from build123d import *

# Parameters (mm, degrees)
SKETCH1_W           = 130
SKETCH1_H           = 15
BOSS_EXTRUDE1_DEPTH = 6
SKETCH2_W           = 90
SKETCH2_H           = 15
BOSS_EXTRUDE2_DEPTH = 22
CUT_EXTRUDE1_REACH  = 134.699
SKETCH3_R           = 3.5
CUT_EXTRUDE2_REACH  = 134.699
SKETCH4_R           = 12.5
CUT_EXTRUDE3_REACH  = 135.825
SKETCH5_R           = 1.625
SKETCH6_R           = 3.5
CUT_EXTRUDE4_DEPTH  = 25.5
FILLET1_R           = 3
FILLET3_R           = 1.5


with BuildPart() as part:
    # Sketch1 → Boss-Extrude1 (new body)
    with BuildSketch(Plane(origin=(0, 0, 0), x_dir=(1, 0, 0), z_dir=(0, 1, 0))):
        with Locations((65, 7.5)):
            Rectangle(SKETCH1_W, SKETCH1_H)
    extrude(amount=BOSS_EXTRUDE1_DEPTH)

    # Sketch2 → Boss-Extrude2 (add)
    with BuildSketch(Plane(origin=(0, 6, 0), x_dir=(1, 0, 0), z_dir=(0, 1, 0))):
        with Locations((65, 7.5)):
            Rectangle(SKETCH2_W, SKETCH2_H)
    extrude(amount=BOSS_EXTRUDE2_DEPTH)

    # Sketch3 → Cut-Extrude1 (cut, up to next)
    with BuildSketch(Plane(origin=(0, 6, 0), x_dir=(1, 0, 0), z_dir=(0, 1, 0)), mode=Mode.PRIVATE) as cut_extrude1_sk1:
        with Locations(Location((10, 7.5, 0), (0, 0, 270))):
            Circle(SKETCH3_R)
    cut_extrude1_tool1 = extrude(cut_extrude1_sk1.sketch, amount=-CUT_EXTRUDE1_REACH, mode=Mode.PRIVATE) & part.part
    # Sketch3 → Cut-Extrude1 (cut, up to next)
    with BuildSketch(Plane(origin=(0, 6, 0), x_dir=(1, 0, 0), z_dir=(0, 1, 0)), mode=Mode.PRIVATE) as cut_extrude1_sk2:
        with Locations(Location((120, 7.5, 0), (0, 0, 270))):
            Circle(SKETCH3_R)
    cut_extrude1_tool2 = extrude(cut_extrude1_sk2.sketch, amount=-CUT_EXTRUDE1_REACH, mode=Mode.PRIVATE) & part.part
    add(cut_extrude1_tool1.solids().sort_by_distance((10, 6, -7.5))[0], mode=Mode.SUBTRACT)
    add(cut_extrude1_tool2.solids().sort_by_distance((120, 6, -7.5))[0], mode=Mode.SUBTRACT)

    # Sketch4 → Cut-Extrude2 (cut, up to next)
    with BuildSketch(Plane(origin=(0, 6, 0), x_dir=(1, 0, 0), z_dir=(0, 1, 0)), mode=Mode.PRIVATE) as cut_extrude2_sk1:
        with Locations((10, 7.5)):
            Circle(SKETCH4_R)
    cut_extrude2_tool1 = extrude(cut_extrude2_sk1.sketch, amount=CUT_EXTRUDE2_REACH, mode=Mode.PRIVATE) & part.part
    # Sketch4 → Cut-Extrude2 (cut, up to next)
    with BuildSketch(Plane(origin=(0, 6, 0), x_dir=(1, 0, 0), z_dir=(0, 1, 0)), mode=Mode.PRIVATE) as cut_extrude2_sk2:
        with Locations((120, 7.5)):
            Circle(SKETCH4_R)
    cut_extrude2_tool2 = extrude(cut_extrude2_sk2.sketch, amount=CUT_EXTRUDE2_REACH, mode=Mode.PRIVATE) & part.part
    add(cut_extrude2_tool1.solids().sort_by_distance((10, 6, -7.5))[0], mode=Mode.SUBTRACT)
    add(cut_extrude2_tool2.solids().sort_by_distance((120, 6, -7.5))[0], mode=Mode.SUBTRACT)

    # Sketch5 → Cut-Extrude3 (cut, up to next)
    with BuildSketch(Plane(origin=(0, 28, 0), x_dir=(1, 0, 0), z_dir=(0, 1, 0)), mode=Mode.PRIVATE) as cut_extrude3_sk1:
        with Locations(Location((42.5, 7.5, 0), (0, 0, 270))):
            Circle(SKETCH5_R)
    cut_extrude3_tool1 = extrude(cut_extrude3_sk1.sketch, amount=-CUT_EXTRUDE3_REACH, mode=Mode.PRIVATE) & part.part
    # Sketch5 → Cut-Extrude3 (cut, up to next)
    with BuildSketch(Plane(origin=(0, 28, 0), x_dir=(1, 0, 0), z_dir=(0, 1, 0)), mode=Mode.PRIVATE) as cut_extrude3_sk2:
        with Locations(Location((87.5, 7.5, 0), (0, 0, 270))):
            Circle(SKETCH5_R)
    cut_extrude3_tool2 = extrude(cut_extrude3_sk2.sketch, amount=-CUT_EXTRUDE3_REACH, mode=Mode.PRIVATE) & part.part
    add(cut_extrude3_tool1.solids().sort_by_distance((42.5, 28, -7.5))[0], mode=Mode.SUBTRACT)
    add(cut_extrude3_tool2.solids().sort_by_distance((87.5, 28, -7.5))[0], mode=Mode.SUBTRACT)

    # Sketch6 → Cut-Extrude4 (cut)
    with BuildSketch(Plane.XZ):
        with Locations(Location((42.5, -7.5, 0), (0, 0, 270))):
            Circle(SKETCH6_R)
        with Locations(Location((87.5, -7.5, 0), (0, 0, 270))):
            Circle(SKETCH6_R)
    extrude(amount=-CUT_EXTRUDE4_DEPTH, mode=Mode.SUBTRACT)

    # Fillet1
    fillet1_edges = [part.edges().sort_by_distance(p)[0] for p in [
        (0, 3, -15),
        (130, 3, -15),
        (130, 3, 0),
        (0, 3, 0),
    ]]
    fillet(fillet1_edges, radius=FILLET1_R)

    # Fillet3
    fillet3_edges = [part.edges().sort_by_distance(p)[0] for p in [
        (20, 17, -15),
        (20, 17, 0),
        (110, 17, 0),
        (110, 17, -15),
    ]]
    fillet(fillet3_edges, radius=FILLET3_R)


solid = part.part
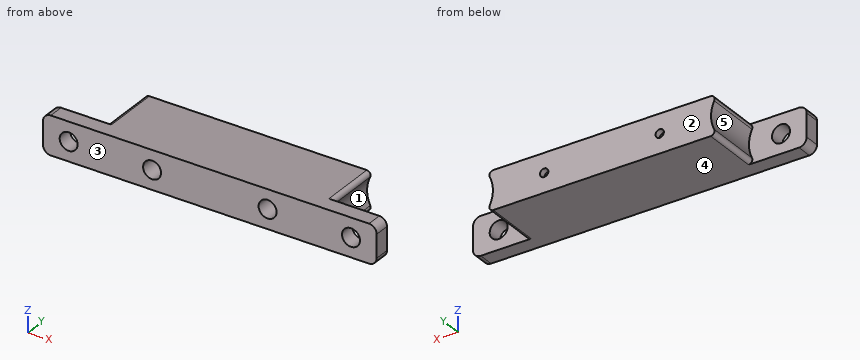
Here's how the part is built. I have some questions about the finished solid (model axes, mm). Face numbers are marked on the shaded views. A direction names the side the tool comes from. Give positions to 0.01 mm unless a question says otherwise; leave off trailing zeros. Loops run counter-clockwise (first coordinate to the right, second up) from the corner with the lowest first, then second, coordinate; pieces in that order, holes last. Notation, with made-up numbers: (42.25, 45) -> (73.25, 45) arc R24 cw to (73.25, 73) -> close; hole circle Ø1 at (87, 57.5). An arc over 180 degrees is marked (long way). One line per item, written item: value.
Q1. I'm going to push flat-ended pins straight in: pin 1 Ø7.5 at (x, z) = (8, -4.5) entering from +Y; pin 2 Ø6 at (y, z) = (24, -4.5) entering from +X; pin 3 Ø5 at (y, z) = (18, -13.5) entering from -X. Where does each tip first touch, or does it pass through?
Answers follow:
pin 1: y = 6
pin 2: x = 108.85
pin 3: x = 21.15
Q2. Suppose I cut it at B-B on x = 42.5. Please give me the cut outline in (y, z) (3 decimals), then the cut area to 3 significant figures.
Answers follow:
outline: (0, -15) -> (28, -15) -> (28, -9.125) -> (25.5, -9.125) -> (25.5, -11) -> (0, -11) -> close; (0, -4) -> (25.5, -4) -> (25.5, -5.875) -> (28, -5.875) -> (28, 0) -> (0, 0) -> close
area: 233 mm^2
Q3. Suppose I cut it at A-A on z = -7.5. State how many separate pieces and enclosed holes the cut face has, then the cut area to 3 significant figures.
Answers follow:
separate pieces: 5
enclosed holes: 0
area: 2,190 mm^2
Q4. We'd pull the mould along Z, two halves only. Please class the marked faces 3, 4 and 5: pulls with the +Z half, pulls with the -Z half, needs draft (parallel to the pull), parting line crosses it, or undercut.
Answers follow:
face 3: needs draft
face 4: pulls with the -Z half
face 5: undercut
Q5. On a 3-axis mill with a long thin cutter (end or side, diameter ignored), from which of +Z, -Z, +X, -X, +Y, -Y can I reach the whole of each face in a straight line? I mean the marked faces 1 and 2. Say none if no direction works.
Answers follow:
face 1: +X, +Y
face 2: +Z, -Z, +X, -X, +Y
Q6. Suppose I cut it at C-C on y = 18.5. Please give me the cut outline in (x, z), then the cut area to 3 significant figures.
Answers follow:
outline: (21.29, -12.86) arc R1.5 ccw to (22.65, -15) -> (107.35, -15) arc R1.5 ccw to (108.71, -12.86) arc R12.5 cw to (108.71, -2.14) arc R1.5 ccw to (107.35, 0) -> (22.65, 0) arc R1.5 ccw to (21.29, -2.14) arc R12.5 cw to start; hole circle Ø7 at (42.5, -7.5); hole circle Ø7 at (87.5, -7.5)
area: 1,220 mm^2
Q7. Suppose I cut it at D-D on y = 3. Please give me the cut outline in (x, z), then the cut area to 3 significant figures.
Answers follow:
outline: (0, -12) arc R3 ccw to (3, -15) -> (127, -15) arc R3 ccw to (130, -12) -> (130, -3) arc R3 ccw to (127, 0) -> (3, 0) arc R3 ccw to (0, -3) -> close; hole circle Ø7 at (10, -7.5); hole circle Ø7 at (42.5, -7.5); hole circle Ø7 at (87.5, -7.5); hole circle Ø7 at (120, -7.5)
area: 1,790 mm^2
Q8. If I drill on line 1 along X through (y, z) = (16, -7.5); line 2 along X through (y, z) = (4.4, -7.5); line 3 along Z through (x, y) = (87.5, 27.45) (3 decimals), over which ranges is the centre line in solid material (lowest first)?
Answers follow:
line 1: 22.5 to 39, 46 to 84, 91 to 107.5
line 2: 0 to 6.5, 13.5 to 39, 46 to 84, 91 to 116.5, 123.5 to 130
line 3: -15 to -9.125, -5.875 to 0
